```python
from build123d import *

# Parameters (mm, degrees)
F0_R      = 40.2650795079
F0_R_2    = 2
F2_DEPTH  = 20
F4_DEPTH  = 69.8
F6_DEPTH  = 25.001
F7_DEPTH  = 5
F8_R      = 2.5
F9_DEPTH  = 14.9319422489
F11_DEPTH = 13


# Not quite as in the source:
# - a feature names something its author has since deleted; it is built from what else it names


with BuildPart() as f2:
    # F0 (on Top) → F2 (new body)
    with BuildSketch(Plane.XY):
        with Locations((-11.4915669638, 7.0636273592)):
            Circle(F0_R)
        with Locations((-26.4915669638, -12.3077432686)):
            Circle(F0_R_2, mode=Mode.SUBTRACT)
        with Locations((3.5084330362, -12.3077432686)):
            Circle(F0_R_2, mode=Mode.SUBTRACT)
        with Locations((-26.4915669638, 26.434997987)):
            Circle(F0_R_2, mode=Mode.SUBTRACT)
        with Locations((3.5084330362, 26.434997987)):
            Circle(F0_R_2, mode=Mode.SUBTRACT)
    extrude(amount=F2_DEPTH)

    # F3 (on Right) → F4 (cut, symmetric)
    with BuildSketch(Plane.YZ):
        Polygon((-43.8041239977, 30.4956686149), (-39.6489202976, 15.9488338977), (68.1266114116, 20.8831354976), (67.6865195207, 30.4956686149), align=None)
    extrude(amount=F4_DEPTH, both=True, mode=Mode.SUBTRACT)

    # F5 (on offset) → F6 (cut, through all)
    with BuildSketch(Plane.XY.offset(25)):
        Polygon((-4.9963764354, 14.8136273592), (-1.5322748203, 8.8136273592), (5.39592841, 8.8136273592), (8.8600300251, 14.8136273592), (5.39592841, 20.8136273592), (-1.5322748203, 20.8136273592), align=None)
        Polygon((-1.5322748203, 5.3136273592), (-4.9963764354, -0.6863726408), (-1.5322748203, -6.6863726408), (5.39592841, -6.6863726408), (8.8600300251, -0.6863726408), (5.39592841, 5.3136273592), align=None)
        Polygon((-14.170220135, -2.8258145228), (-17.6343217501, -8.8258145228), (-14.170220135, -14.8258145228), (-7.2420169047, -14.8258145228), (-3.7779152896, -8.8258145228), (-7.2420169047, -2.8258145228), align=None)
        Polygon((-27.5721969216, 4.890474733), (-31.0362985367, -1.109525267), (-27.5721969216, -7.109525267), (-20.6439936913, -7.109525267), (-17.1798920761, -1.109525267), (-20.6439936913, 4.890474733), align=None)
        Polygon((-7.1614399449, 14.5636273592), (-15.8216939827, 14.5636273592), (-20.1518210017, 7.0636273592), (-15.8216939827, -0.4363726408), (-7.1614399449, -0.4363726408), (-2.831312926, 7.0636273592), align=None)
        Polygon((-27.6414862443, 20.3495556396), (-31.1520113303, 14.3765987822), (-27.7345414991, 8.3499164484), (-20.8065465819, 8.296190972), (-17.2960214958, 14.2691478294), (-20.7134913271, 20.2958301632), align=None)
        Polygon((-14.0889966993, 28.28301467), (-17.5530983144, 22.28301467), (-14.0889966993, 16.28301467), (-7.160793469, 16.28301467), (-3.6966918539, 22.28301467), (-7.160793469, 28.28301467), align=None)
    extrude(amount=-F6_DEPTH, mode=Mode.SUBTRACT)

    # F7 (cut): a face of the model
    f7_faces = [f2.faces().sort_by_distance(p)[0] for p in [
        (-50.6177780411, 7.0636273592, 0),
    ]]
    extrude(f7_faces, amount=-F7_DEPTH, mode=Mode.SUBTRACT)

    # F8 (on face) → F9 (cut, through all)
    with BuildSketch(Plane(origin=(0, 0, 5), x_dir=(1, 0, 0), z_dir=(0, 0, -1))):
        with Locations((14.8332985118, 10.2885384113)):
            Circle(F8_R)
        with Locations((14.8332985118, -24.3908837438)):
            Circle(F8_R)
        with Locations((-37.8164324394, -24.4157931297)):
            Circle(F8_R)
        with Locations((-37.8164324394, 10.2885384113)):
            Circle(F8_R)
    extrude(amount=-F9_DEPTH, mode=Mode.SUBTRACT)

    # F10 (on offset) → F11 (cut)
    with BuildSketch(Plane.XY.offset(25)):
        Polygon((19.2582985118, -12.8433133524), (19.2582985118, -7.7337634701), (14.8332985118, -5.1789885289), (10.4082985118, -7.7337634701), (10.4082985118, -12.8433133524), (14.8332985118, -15.3980882936), align=None)
        Polygon((19.2582985118, 21.8361088026), (19.2582985118, 26.9456586849), (14.8332985118, 29.5004336261), (10.4082985118, 26.9456586849), (10.4082985118, 21.8361088026), (14.8332985118, 19.2813338614), align=None)
        Polygon((-33.3914324394, 21.8610181886), (-33.3914324394, 26.9705680709), (-37.8164324394, 29.5253430121), (-42.2414324394, 26.9705680709), (-42.2414324394, 21.8610181886), (-37.8164324394, 19.3062432474), align=None)
        Polygon((-33.3914324394, -12.8433133524), (-33.3914324394, -7.7337634701), (-37.8164324394, -5.1789885289), (-42.2414324394, -7.7337634701), (-42.2414324394, -12.8433133524), (-37.8164324394, -15.3980882936), align=None)
    extrude(amount=-F11_DEPTH, mode=Mode.SUBTRACT)


solid = f2.part
```
Check sheet for the modelled part. Datum: model origin and axes. Units: mm. A direction names the side the tool comes from. Coordinates: 2 decimals unless noted, no trailing zeros. Order: outer loops, then holes, each group sorted by start corner. A loop starts at its lowest first (then second) coordinate and runs counter-clockwise, first axis right, second up. Notation, with made-up numbers: M 49.5,42 L 80.5,42 A13 cw 80.5,60 Z; hole C 23.25,29 d1. An arc over 180 degrees is marked long. Write each question's results on one line, items separated by ' | '. Start each with the question number.
1. Access from +Z, -Z, +X, -X, +Y, -Y to the whole of each face (thin tool, end or side, straight path). Record for faces 1 (the face through (-17.956, 10.866, 11.809)), 2 (the face through (-33.391, 24, 16)).
2. Cross-section at D-D on y = -17. Record the cut outline in (x, z), and give its area (3 significant figures).
3. Material ranges on probe 1 along Y at (x, z) = (-12, 12.5); probe 2 along Y at (x, z) = (-8.5, 17.5); probe 3 along X at (y, z) = (18, 7.75), recorded low to high.
4. Mould release check, pull along Y, two halves, no side actions. Record for faces 3 (the face through (-16.733, 46.986, 12.383)), 4 (the face through (-42.241, 24, 16)), 5 (the face through (-12, -1, 5)): +Y half, -Y half, draft (parallel to the pull), parting line (faces both ways), or undercut.
5. Cross-section at C-C on z = 14.5. State how many separate pieces and enclosed holes the cut face has, and give its area (3 significant figures).
6. Cross-section at B-B on y = 12. Record the cut outline in (x, z).
7. Cross-section at A-A on x = 6.5. Record the cut outline in (y, z).
8. Go/stop test with flat-tipped pins: P1, Ø1.5, axis at y = 24.5, z = 14, coming from the +X side; P2, Ø5.5, axis at x = -11.5, z = 15, coming from the +Y side; P3, Ø3.5, axis at x = 2.5, z = 11.5, coming from the +Y side. Record where each tip stops, or that it passes through.
Checks:
1) face 1: +Z, -Z | face 2: +Z
2) outline: M -43.77,5 L 20.79,5 L 20.79,16.99 L -43.77,16.99 Z | area: 774 mm²
3) probe 1: y = -33.2 to -14.83, -2.83 to -0.44, 14.56 to 16.28, 28.28 to 47.33 | probe 2: y = -2.83 to -0.44, 14.56 to 16.28, 28.28 to 47.22 | probe 3: x = -50.24 to -29.02, -19.41 to -15.08, -6.17 to -3.16, 7.02 to 27.26
4) face 3: parting line | face 4: undercut | face 5: draft
5) separate pieces: 1 | enclosed holes: 15 | area: 3,830 mm²
6) outline: M -51.45,5 L -29.8,5 L -29.8,18.31 L -51.45,18.31 Z; M -18.63,5 L -17.3,5 L -17.3,18.31 L -18.63,18.31 Z; M -5.68,5 L -3.37,5 L -3.37,18.31 L -5.68,18.31 Z; M 7.24,5 L 28.47,5 L 28.47,18.31 L 7.24,18.31 Z
7) outline: M -28.96,5 L -4.77,5 L -4.77,17.55 L -28.96,16.44 Z; M 3.4,5 L 10.73,5 L 10.73,18.26 L 3.4,17.92 Z; M 18.9,5 L 43.09,5 L 43.09,19.74 L 18.9,18.63 Z
8) P1: stops at x = 25.15 | P2: stops at y = 47.33 | P3: stops at y = 45.42
